The model under review builds one solid part; all positions refer to its coordinate system, in mm. Round coordinates to 2 decimals unless told otherwise and drop trailing zeros. Write each loop counter-clockwise with the first axis right and the second up, starting at its lowest first coordinate (ties: lowest second). Pieces come first, ordered by that corner, then holes. Notation, with made-up numbers: (37.5, -31.75) -> (92.5, -31.75) arc R24 cw to (92.5, -15.75) -> close; hole circle Ø5 at (50.25, 69.25). An arc over 180 degrees is marked (long way). Answer in a Markdown table with one row per item. Add a question column.
```python
from build123d import *

# Parameters (mm, degrees)
SKETCH_R  = 4
PAD_DEPTH = 12


with BuildPart() as part:
    # Sketch → Pad (new body)
    with BuildSketch(Plane.XY):
        with BuildLine():
            ThreePointArc((-4, -14.456832), (0, -15), (4, -14.456832))
            Line((32.478293, -6.577294), (4, -14.456832))
            ThreePointArc((32.478293, -6.577294), (37.040054, 0.307444), (31.867844, 6.746196))
            Line((31.867844, 6.746196), (4, 14.456832))
            ThreePointArc((4, 14.456832), (0, 15), (-4, 14.456832))
            Line((-31.75668, 6.775993), (-4, 14.456832))
            ThreePointArc((-31.75668, 6.775993), (-36.999768, 0.056933), (-31.866667, -6.746522))
            Line((-31.866667, -6.746522), (-4, -14.456832))
        make_face()
        with Locations((-30, 0)):
            Circle(SKETCH_R, mode=Mode.SUBTRACT)
        with Locations((30, 0)):
            Circle(SKETCH_R, mode=Mode.SUBTRACT)
    extrude(amount=PAD_DEPTH)


solid = part.part
```
1. Insertion check: pin 1 Ø1 at (x, z) = (5, 7) entering from +Y; pin 2 Ø6 at (y, z) = (9, 2) entering from +X; pin 3 Ø4 at (x, z) = (17, 5.5) entering from -Y. Each pin has a flat end and moves straight along its axis. Give the tip position at first contact, or say it passes through.
2. For L1, parallel to X at y = 2.5, z = 7; L2, parallel to X at y = 2.25, z = 5.25; L3, parallel to Y at x = 30, z = 8, list the stretches that pass through material, from the lowest coordinate up.
3. Add section A-A on y = 2.5. Write out the cut boundary in (x, z).
4. Add section B-B on z = 4.5. Write out the cut boundary in (x, y).
5. Add section C-C on x = 30. Write out the cut boundary in (y, z).
6. Mouldability with a two-part tool opening along X and no side actions: class faces 1 (the cylindrical face through (26.8, -2.4, 5.9)), 2 (the flat face through (-18.128, -10.548, 5.916)), 3 (the cylindrical face through (-33.2, -2.4, 5.9)), 4 (the flat face through (0, 0, 12)) as pulls with the +X half, pulls with the -X half, needs draft (parallel to the pull), parting line crosses it, or undercut.
Filled in:
| question | item | result |
|---|---|---|
| 1 | pin 1 | y = 14.32 |
| 1 | pin 2 | x = 33.63 |
| 1 | pin 3 | y = -11.41 |
| 2 | L1 | -36.54 to -33.12, -26.88 to 26.88, 33.12 to 36.58 |
| 2 | L2 | -36.63 to -33.31, -26.69 to 26.69, 33.31 to 36.67 |
| 2 | L3 | -7.26 to -4, 4 to 7.26 |
| 3 | outline | (-36.54, 0) -> (-33.12, 0) -> (-33.12, 12) -> (-36.54, 12) -> close; (-26.88, 0) -> (26.88, 0) -> (26.88, 12) -> (-26.88, 12) -> close; (33.12, 0) -> (36.58, 0) -> (36.58, 12) -> (33.12, 12) -> close |
| 4 | outline | (-31.87, -6.75) -> (-4, -14.46) arc R15 ccw to (4, -14.46) -> (32.48, -6.58) arc R7 ccw to (31.87, 6.75) -> (4, 14.46) arc R15 ccw to (-4, 14.46) -> (-31.76, 6.78) arc R7 ccw to start; hole circle Ø8 at (-30, 0); hole circle Ø8 at (30, 0) |
| 5 | outline | (-7.26, 0) -> (-4, 0) -> (-4, 12) -> (-7.26, 12) -> close; (4, 0) -> (7.26, 0) -> (7.26, 12) -> (4, 12) -> close |
| 6 | face 1 | undercut |
| 6 | face 2 | pulls with the -X half |
| 6 | face 3 | undercut |
| 6 | face 4 | needs draft |
